Read the model definition and answer for the solid it produces. Units are mm, in the model's axes. Round coordinates to 2 decimals unless told otherwise and drop trailing zeros. Loops run counter-clockwise (first coordinate to the right, second up) from the corner with the lowest first, then second, coordinate; pieces in that order, holes last. Notation, with made-up numbers: M 86,47 L 130,47 A20 ccw 130,54 Z; hole C 59.5,28.5 d4. An arc over 180 degrees is marked long. Write each question's results on one line, items separated by ' | '.
from build123d import *

# Parameters (mm, degrees)
SKETCH1_R           = 19.685
SKETCH1_R_2         = 2.499995
BOSS_EXTRUDE1_DEPTH = 3.175


with BuildPart() as part:
    # Sketch1 → Boss-Extrude1 (new body)
    with BuildSketch(Plane(origin=(0, 0, 0), x_dir=(1, 0, 0), z_dir=(0, 1, 0))):
        with BuildLine():
            Line((-13.993314597, 28.4999938), (-25.9599938, 28.4999938))
            ThreePointArc((-25.9599938, 28.4999938), (-27.756045024, 27.756045024), (-28.4999938, 25.9599938))
            Line((-28.4999938, 25.9599938), (-28.4999938, 13.993314597))
            Line((-28.4999938, 13.993314597), (-28.4999938, -13.993314597))
            Line((-28.4999938, -13.993314597), (-28.4999938, -25.9599938))
            ThreePointArc((-28.4999938, -25.9599938), (-27.756045024, -27.756045024), (-25.9599938, -28.4999938))
            Line((-25.9599938, -28.4999938), (-13.993314597, -28.4999938))
            Line((-13.993314597, -28.4999938), (13.993314597, -28.4999938))
            Line((13.993314597, -28.4999938), (25.9599938, -28.4999938))
            ThreePointArc((25.9599938, -28.4999938), (27.756045024, -27.756045024), (28.4999938, -25.9599938))
            Line((28.4999938, -25.9599938), (28.4999938, -13.993314597))
            Line((28.4999938, -13.993314597), (28.4999938, 13.993314597))
            Line((28.4999938, 13.993314597), (28.4999938, 25.9599938))
            ThreePointArc((28.4999938, 25.9599938), (27.756045024, 27.756045024), (25.9599938, 28.4999938))
            Line((25.9599938, 28.4999938), (13.993314597, 28.4999938))
            Line((13.993314597, 28.4999938), (-13.993314597, 28.4999938))
        make_face()
        Circle(SKETCH1_R, mode=Mode.SUBTRACT)
        with Locations((-23.5000038, 23.5000038)):
            Circle(SKETCH1_R_2, mode=Mode.SUBTRACT)
        with Locations((23.5000038, 23.5000038)):
            Circle(SKETCH1_R_2, mode=Mode.SUBTRACT)
        with Locations((23.5000038, -23.5000038)):
            Circle(SKETCH1_R_2, mode=Mode.SUBTRACT)
        with Locations((-23.5000038, -23.5000038)):
            Circle(SKETCH1_R_2, mode=Mode.SUBTRACT)
    extrude(amount=BOSS_EXTRUDE1_DEPTH)


solid = part.part
Item 1: The part is cut by section C-C (x = 0). Determine the outline of the cut face in (y, z) (3 decimals), plus the area to 3 significant figures.
Outcome:
outline: M 0,-28.5 L 3.175,-28.5 L 3.175,-19.685 L 0,-19.685 Z; M 0,19.685 L 3.175,19.685 L 3.175,28.5 L 0,28.5 Z | area: 56.0 mm2
Item 2: Straight lines are drawn through the part: line 1 (X direction, y = 2.3, z = -23.5); line 2 (Z direction, x = 24.5, y = 0.65); line 3 (X direction, y = 0.9, z = 25). For each, find the intervals that lie inside material, in ascending order.
Outcome:
line 1: x = -28.5 to -26, -21 to 21, 26 to 28.5 | line 2: z = -28.5 to -25.79, -21.21 to 21.21, 25.79 to 28.5 | line 3: x = -28.5 to -25.5, -21.5 to 21.5, 25.5 to 28.5
Item 3: The mould has two halves that part along Z. Classify faces 1 (the face through (27.776, 1.565, -27.736)), 2 (the face through (-7, 3.175, -19)), 3 (the face through (24.84, 1.57, -25.61)): pulls with the +Z half, pulls with the -Z half, needs draft (parallel to the pull), parting line crosses it, or undercut.
Outcome:
face 1: pulls with the -Z half | face 2: needs draft | face 3: undercut
Item 4: The part is cut by section B-B (y = 1.75). Determine the outline of the cut face in (x, z) (3 decimals), plus the area to 3 significant figures.
Outcome:
outline: M -28.5,-25.96 A2.54 ccw -25.96,-28.5 L 25.96,-28.5 A2.54 ccw 28.5,-25.96 L 28.5,25.96 A2.54 ccw 25.96,28.5 L -25.96,28.5 A2.54 ccw -28.5,25.96 Z; hole C -23.5,-23.5 d5; hole C -23.5,23.5 d5; hole C 0,0 d39.37; hole C 23.5,-23.5 d5; hole C 23.5,23.5 d5 | area: 1,950 mm2
Item 5: The part is cut by section A-A (z = 0). Determine the outline of the cut face in (x, y) (3 decimals), plus the area to 3 significant figures.
Outcome:
outline: M -28.5,0 L -19.685,0 L -19.685,3.175 L -28.5,3.175 Z; M 19.685,0 L 28.5,0 L 28.5,3.175 L 19.685,3.175 Z | area: 56.0 mm2
Item 6: Flat-ended cylindrical pins translate along their axes: pin 1 (6.5 mm diameter, centred on x = 23.5, z = -23.5, fed in from +Y) (3 decimals); pin 2 (3 mm diameter, centred on x = -23.5, z = 23.5, fed in from -Y) (1 decimal). Find the tip coordinate at first contact, or state that the pin passes through.
Outcome:
pin 1: stops at y = 3.175 | pin 2: passes through
